Read the model definition and answer for the solid it produces. Units are mm, in the model's axes. A direction names the side the tool comes from. Coordinates: 2 decimals unless noted, no trailing zeros. Loops run counter-clockwise (first coordinate to the right, second up) from the corner with the lowest first, then second, coordinate; pieces in that order, holes last. Notation, with made-up numbers: M 81.5,-17 L 119.5,-17 A31 ccw 119.5,12 Z; hole C 58,-2 d8. An arc over 180 degrees is marked long. Use one line per item in the form item = value. Start each with the question number.
1. Find the intervals of material crossed by probe 1 along Y at (x, z) = (0, -24); probe 2 along Y at (x, z) = (804, -546), in increasing order. Write a range as [from, to].
2. The part is cut by section A-A (y = -71.5). Give the vertices of the cut face in (x, z), plus the area to 3 significant figures.
3. The part is cut by section D-D (z = -312.5). Give the vertices of the cut face in (x, y).
4. A tool of negligible diameter and unlimited length cuts with its end or side. For faces 1 (the flat face through (2666, -52, -31.75)), 2 (the cylindrical face through (1.396, 63.485, -15.653)), from which of +Z, -Z, +X, -X, +Y, -Y can it reach the whole face along a straight path? Write none if from no direction.
5. The part is cut by section C-C (x = 629). Give the vertices of the cut face in (y, z), plus the area to 3 significant figures.
6. For a pull along Y with two mould halves and no side action, classify faces 3 (the flat face through (2730.5, -185, -313)), 4 (the cylindrical face through (-6.883, -30.995, -15.653)), 5 (the cylindrical face through (2635.28, 1.4, -15.65)), 6 (the cylindrical face through (2668.396, 63.485, -15.653)) as released by +Y, released by -Y, zero draft, split by the parting line, or undercut.
7. A flat-ended cylindrical pin translates along its axis: pin 1 (2 mm diameter, centred on x = 278, z = -493, fed in from +Y). Find the tip coordinate at first contact, or state that the pin passes through.
8. The part is cut by section B-B (x = 2667). Give the vertices of the cut face in (y, z), plus the area to 3 significant figures.
from build123d import *

# Parameters (mm, degrees)
SKETCH1_R           = 63.5
SKETCH1_W           = 127
SKETCH1_H           = 127
BOSS_EXTRUDE1_DEPTH = 31.75
SKETCH2_W           = 2794
SKETCH2_H           = 127
BOSS_EXTRUDE2_DEPTH = 635
SKETCH3_R           = 31.75
CUT_EXTRUDE1_DEPTH  = 2815.848352931


with BuildPart() as part:
    # Sketch1 → Boss-Extrude1 (new body)
    with BuildSketch(Plane.XY):
        Circle(SKETCH1_R)
        with Locations((2667, 0)):
            Circle(SKETCH1_R)
        with Locations((0, -63.5)):
            Rectangle(SKETCH1_W, SKETCH1_H)
        with Locations((2667, -63.5)):
            Rectangle(SKETCH1_W, SKETCH1_H)
    extrude(amount=-BOSS_EXTRUDE1_DEPTH)

    # Sketch2 → Boss-Extrude2 (add)
    with BuildSketch(Plane.XY):
        with Locations((1333.5, -190.5)):
            Rectangle(SKETCH2_W, SKETCH2_H)
    extrude(amount=-BOSS_EXTRUDE2_DEPTH)

    # Sketch3 → Cut-Extrude1 (cut, through all)
    with BuildSketch(Plane.XY):
        Circle(SKETCH3_R)
        with Locations((2667, 0)):
            Circle(SKETCH3_R)
    extrude(amount=-CUT_EXTRUDE1_DEPTH, mode=Mode.SUBTRACT)


solid = part.part
Computed values:
q1.probe_1 = [-254, -31.75], [31.75, 63.5]
q1.probe_2 = [-254, -127]
q2.outline = M -63.5,-31.75 L 63.5,-31.75 L 63.5,0 L -63.5,0 Z; M 2603.5,-31.75 L 2730.5,-31.75 L 2730.5,0 L 2603.5,0 Z
q2.area = 8,060 mm²
q3.outline = M -63.5,-254 L 2730.5,-254 L 2730.5,-127 L -63.5,-127 Z
q4.face_1 = -Z, +X, -X, +Y
q4.face_2 = +Z, -Z, +Y
q5.outline = M -254,-635 L -127,-635 L -127,0 L -254,0 Z
q5.area = 80,600 mm²
q6.face_3 = zero draft
q6.face_4 = undercut
q6.face_5 = undercut
q6.face_6 = released by +Y
q7.pin_1 = -127
q8.outline = M -254,-635 L -127,-635 L -127,-31.75 L -31.75,-31.75 L -31.75,0 L -254,0 Z; M 31.75,-31.75 L 63.5,-31.75 L 63.5,0 L 31.75,0 Z
q8.area = 84,700 mm²
